Part model, mm, in its own coordinate system. A direction names the side the tool comes from. Give positions to 0.01 mm unless a question says otherwise; leave off trailing zeros. Order: outer loops, then holes, each group sorted by start corner. A loop starts at its lowest first (then second) coordinate and runs counter-clockwise, first axis right, second up.
1. Slice it at B-B on x = 2.25. List the corners of the cut face in (y, z), and give its area (3 significant figures).
2. Slice it at A-A on y = 0. List the corners of the cut face in (x, z), and give its area (3 significant figures).
3. Drop flat-ended pins along their axis: pin 1 Ø0.5 at (x, y) = (2, 0) entering from -Z; pin 2 Ø0.7 at (x, y) = (6, 0) entering from -Z; pin 3 Ø1 at (x, y) = (5.5, -1) entering from +Z; pin 4 Ø1.5 at (x, z) = (3.5, 1.5) entering from -Y. Give the stop position or say it passes through.
4. Slice it at C-C on z = -1.85. List the corners of the cut face in (x, y).
5. Slice it at D-D on y = 1. List the corners of the cut face in (x, z).
6. Probe line 1 (Z direction, x = 7.5, y = -0.1); line 2 (X direction, y = 0, z = 0.5); line 3 (X direction, y = -0.15, z = 0.8). List the from-to ranges inside material, lowest first.
7. Which spindle directions (+Z, -Z, +X, -X, +Y, -Y) get a long thin tool onto all of the face, cutting with end or side? Do faces 1 (the flat face through (-1.6, 0.3, -0.3)), 2 (the flat face through (1, 0, 2.54)), 3 (the flat face through (1, 0, 0)), 4 (the flat face through (-1.6, -0.3, -0.3)). Say none if no direction does.
from build123d import *

# Parameters (mm, degrees)
PLASTIC_DEPTH = 2.54
CONTACT_DEPTH = 0.3
CHAMFER1_SIZE = 0.1


with BuildPart() as part:
    # Sketch1 → Plastic (new body)
    with BuildSketch(Plane(origin=(0, 0, 0), x_dir=(0, 0, -1), z_dir=(1, 0, 0))):
        Polygon((-2.04, 1.27), (-0.5, 1.27), (0, 0.77), (0, -0.77), (-0.5, -1.27), (-2.04, -1.27), (-2.54, -0.77), (-2.54, 0.77), align=None)
    extrude(amount=PLASTIC_DEPTH)

    # Sketch2 → Contact (add, symmetric)
    with BuildSketch(Plane(origin=(0, 0, 0), x_dir=(1, 0, 0), z_dir=(0, 1, 0))):
        with BuildLine():
            Line((-1.86, 3.36), (-1.86, -0.67))
            ThreePointArc((-1.86, -0.67), (-1.596396103, -1.306396103), (-0.96, -1.57))
            Line((-0.96, -1.57), (8.9, -1.57))
            Line((8.9, -1.57), (8.9, -0.97))
            Line((8.9, -0.97), (-0.96, -0.97))
            ThreePointArc((-0.96, -0.97), (-1.172132034, -0.882132034), (-1.26, -0.67))
            Line((-1.26, -0.67), (-1.26, 3.36))
            Line((-1.26, 3.36), (-1.86, 3.36))
        make_face()
    extrude(amount=CONTACT_DEPTH, both=True)

    # Chamfer1
    chamfer1_edges = [part.edges().sort_by_distance(p)[0] for p in [
        (8.9, 0, 0.97),
        (8.9, 0.3, 1.27),
        (-1.56, -0.3, -3.36),
        (-1.26, 0, -3.36),
        (-1.86, 0, -3.36),
        (8.9, -0.3, 1.27),
        (8.9, 0, 1.57),
        (-1.56, 0.3, -3.36),
    ]]
    chamfer(chamfer1_edges, length=CHAMFER1_SIZE)


solid = part.part
Data:
1. outline: (-1.27, 0.5) - (-0.77, 0) - (0.77, 0) - (1.27, 0.5) - (1.27, 2.04) - (0.77, 2.54) - (-0.77, 2.54) - (-1.27, 2.04) - close
1. area: 5.95 mm2
2. outline: (-1.86, -3.26) - (-1.76, -3.36) - (-1.36, -3.36) - (-1.26, -3.26) - (-1.26, 0.67) arc R0.3 cw to (-0.96, 0.97) - (0, 0.97) - (0, 0) - (2.54, 0) - (2.54, 0.97) - (8.8, 0.97) - (8.9, 1.07) - (8.9, 1.47) - (8.8, 1.57) - (2.54, 1.57) - (2.54, 2.54) - (0, 2.54) - (0, 1.57) - (-0.96, 1.57) arc R0.9 ccw to (-1.86, 0.67) - close
2. area: 13.8 mm2
3. pin 1: stops at z = 0
3. pin 2: stops at z = 0.97
3. pin 3: passes through
3. pin 4: stops at y = -0.3
4. outline: (-1.86, -0.3) - (-1.26, -0.3) - (-1.26, 0.3) - (-1.86, 0.3) - close
5. outline: (0, 0.23) - (2.54, 0.23) - (2.54, 2.31) - (0, 2.31) - close
6. line 1: z = 0.97 to 1.57
6. line 2: x = -1.86 to -1.26, 0 to 2.54
6. line 3: x = -1.85 to -1.23, 0 to 2.54
7. face 1: +Z, -Z, -X, +Y
7. face 2: +Z, +X, -X, +Y, -Y
7. face 3: -Z, +X, +Y, -Y
7. face 4: +Z, -Z, -X, -Y
